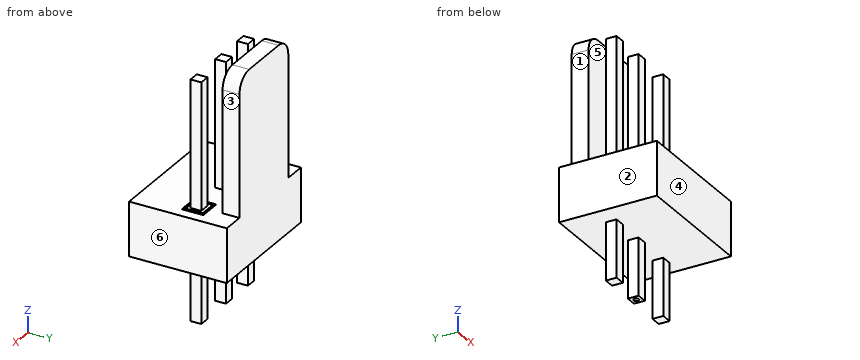
from build123d import *

# Parameters (mm, degrees)
SKETCH_2_W          = 7.62
SKETCH_2_H          = 5.8
EXTRUDE_1_DEPTH     = 3.2
SKETCH_3_W          = 5.02
SKETCH_3_H          = 1
EXTRUDE_4_DEPTH     = 8.2
FILLET_1_R          = 1
SKETCH_1_W          = 0.64
SKETCH_1_H          = 0.64
EXTRUDE_5_DEPTH     = 10.7
SKETCH_1_3_W        = 0.64
SKETCH_1_3_H        = 0.64
EXTRUDE_6_DEPTH     = 3.4
SKETCH_4_W          = 1.33797987
SKETCH_4_H          = 1.281998632
SKETCH_4_W_2        = 1.037697307
SKETCH_4_H_2        = 1.007056107
CUT_EXTRUDE_1_DEPTH = 0.1
SKETCH_5_R          = 0.155933924
CUT_EXTRUDE_2_DEPTH = 2


with BuildPart() as part:
    # Эскиз2 → Вытянуть1 (new body)
    with BuildSketch(Plane.XY):
        with Locations((-2.51, -0.5)):
            Rectangle(SKETCH_2_W, SKETCH_2_H)
    extrude(amount=EXTRUDE_1_DEPTH)

    # Эскиз3 → Вытянуть4 (add)
    with BuildSketch(Plane.XY.offset(3.2)):
        with Locations((-2.51, 1.9)):
            Rectangle(SKETCH_3_W, SKETCH_3_H)
    extrude(amount=EXTRUDE_4_DEPTH)

    # Скругление1
    fillet_1_edges = [part.edges().sort_by_distance(p)[0] for p in [
        (0, 1.9, 11.4),
        (-5.02, 1.9, 11.4),
    ]]
    fillet(fillet_1_edges, radius=FILLET_1_R)

    # Эскиз1 → Вытянуть5 (add)
    with BuildSketch(Plane.XY):
        Rectangle(SKETCH_1_W, SKETCH_1_H)
        with Locations((-2.54, 0)):
            Rectangle(SKETCH_1_W, SKETCH_1_H)
        with Locations((-4.798195283, 0)):
            Rectangle(SKETCH_1_W, SKETCH_1_H)
    extrude(amount=EXTRUDE_5_DEPTH)

    # Эскиз1<3> → Вытянуть6 (add)
    with BuildSketch(Plane.XY):
        Rectangle(SKETCH_1_3_W, SKETCH_1_3_H)
        with Locations((-2.54, 0)):
            Rectangle(SKETCH_1_3_W, SKETCH_1_3_H)
        with Locations((-4.798195283, 0)):
            Rectangle(SKETCH_1_3_W, SKETCH_1_3_H)
    extrude(amount=-EXTRUDE_6_DEPTH)

    # Эскиз4 → Вырез-Вытянуть1 (cut)
    with BuildSketch(Plane(origin=(-0.765860317, 1.721958185, 3.2), x_dir=(1, 0, 0), z_dir=(0, 0, 1))):
        with Locations((0.761284953, -1.723378162)):
            Rectangle(SKETCH_4_W, SKETCH_4_H)
        with Locations((0.75264785, -1.718405131)):
            Rectangle(SKETCH_4_W_2, SKETCH_4_H_2, mode=Mode.SUBTRACT)
    extrude(amount=-CUT_EXTRUDE_1_DEPTH, mode=Mode.SUBTRACT)

    # Эскиз5 → Вырез-Вытянуть2 (cut)
    with BuildSketch(Plane(origin=(0, 0, -3.4), x_dir=(-1, 0, 0), z_dir=(0, 0, -1))):
        with Locations((2.54, 0)):
            Circle(SKETCH_5_R)
    extrude(amount=-CUT_EXTRUDE_2_DEPTH, mode=Mode.SUBTRACT)


solid = part.part
Work out the finished part from the listing and answer in its coordinate system (mm). Face numbers are marked on the shaded views. A direction names the side the tool comes from. Round coordinates to 2 decimals unless told otherwise and drop trailing zeros. Loops run counter-clockwise (first coordinate to the right, second up) from the corner with the lowest first, then second, coordinate; pieces in that order, holes last. Notation, with made-up numbers: (40.25, 32) - (55.25, 32) arc R20 cw to (55.25, 66) - close; hole circle Ø10 at (84.5, -5.5). An arc over 180 degrees is marked (long way). Use one line per item in the form item = value. Start each with the question number.
(1) Determine the mould class of the marked faces 4, 5 and 6 for opening direction Y: +Y half, -Y half, draft (parallel to the pull), parting line (faces both ways), or undercut.
(2) Find section C-C on x = -2.54. Determine the outline of the cut face in (y, z).
(3) Consider line 1 (Y direction, x = -2.54, z = -2.85); line 2 (Z direction, x = -3.5, y = -1.2); line 3 (Y direction, x = -3.25, z = 9.5). Determine where each line is inside the solid, lowest interval first.
(4) Flat-ended cylindrical pins translate along their axes: P1, Ø0.7, axis at y = 0, z = 6.5, coming from the -X side; P2, Ø0.5, axis at x = -4.5, y = 0, coming from the +Z side; P3, Ø0.7, axis at x = -2.5, z = -2, coming from the -Y side. Find the tip coordinate at first contact, or state that the pin passes through.
(5) Which of the six approach directions +Z, -Z, +X, -X, +Y, -Y give full straight-line access (tool end or side, diameter ignored) to the marked faces 1, 2 and 3?
(6) Find section A-A on z = -0.5. Determine the outline of the cut face in (x, y).
(7) Find section D-D on y = -2.65. Determine the outline of the cut face in (x, z).
(8) Find section B-B on z = 8.25. Determine the outline of the cut face in (x, y), and give its area (3 significant figures).
Answer list:
q1.face_4 = -Y half
q1.face_5 = undercut
q1.face_6 = draft
q2.outline = (-3.4, 0) - (-0.32, 0) - (-0.32, -3.4) - (-0.16, -3.4) - (-0.16, -1.4) - (0.16, -1.4) - (0.16, -3.4) - (0.32, -3.4) - (0.32, 0) - (2.4, 0) - (2.4, 11.4) - (1.4, 11.4) - (1.4, 3.2) - (0.32, 3.2) - (0.32, 10.7) - (-0.32, 10.7) - (-0.32, 3.2) - (-3.4, 3.2) - close
q3.line_1 = -0.32 to -0.16, 0.16 to 0.32
q3.line_2 = 0 to 3.2
q3.line_3 = 1.4 to 2.4
q4.P1 = -5.12
q4.P2 = 10.7
q4.P3 = -0.32
q5.face_1 = +Z, -X, +Y
q5.face_2 = +Z, -Z, -X, +Y, -Y
q5.face_3 = +Z, +X, +Y
q6.outline = (-5.12, -0.32) - (-4.48, -0.32) - (-4.48, 0.32) - (-5.12, 0.32) - close; (-2.86, -0.32) - (-2.22, -0.32) - (-2.22, 0.32) - (-2.86, 0.32) - close; (-0.32, -0.32) - (0.32, -0.32) - (0.32, 0.32) - (-0.32, 0.32) - close
q7.outline = (-6.32, 0) - (1.3, 0) - (1.3, 3.2) - (-6.32, 3.2) - close
q8.outline = (-5.12, -0.32) - (-4.48, -0.32) - (-4.48, 0.32) - (-5.12, 0.32) - close; (-5.02, 1.4) - (0, 1.4) - (0, 2.4) - (-5.02, 2.4) - close; (-2.86, -0.32) - (-2.22, -0.32) - (-2.22, 0.32) - (-2.86, 0.32) - close; (-0.32, -0.32) - (0.32, -0.32) - (0.32, 0.32) - (-0.32, 0.32) - close
q8.area = 6.25 mm^2
